Here's how the part is built. I have some questions about the finished solid (model axes, mm). Face numbers are marked on the shaded views. A direction names the side the tool comes from. Give positions to 0.01 mm unless a question says otherwise; leave off trailing zeros. Loops run counter-clockwise (first coordinate to the right, second up) from the corner with the lowest first, then second, coordinate; pieces in that order, holes last.
Q1. If we section it at A-A (x = 15): Please give me the cut outline in (y, z), plus the area to 3 significant figures.
Q2. I need wall thicknesses on line 1 (Y direction, x = 0, z = -38); line 2 (Y direction, x = -0.5, z = -27); line 3 (Y direction, x = -32.5, z = -31.5). Which ranges of each line are inside material? Lowest first, please.
Q3. If we section it at C-C (z = -11): Please give me the cut outline in (x, y), plus the area to 3 significant figures.
Q4. If we section it at D-D (x = 0): Give the number of separate pieces and of enclosed holes in the cut face, plus the area to 3 significant figures.
Q5. If we section it at B-B (z = -26): Please give me the cut outline in (x, y).
Q6. Will these pins go through, and if not, where does the flat tip stop? P1, Ø1, axis at x = -25, y = 13.5, coming from the -Z side; P2, Ø9, axis at x = 6.47, y = 42.54, coming from the -Z side; P3, Ø1.9, axis at y = 102.5, z = -41, coming from the +X side.
Q7. For the marked faces 4, 5 and 6, which set-ups out of +Z, -Z, +X, -X, +Y, -Y let a thin tool reach every point of the face, with its end or its side?
Q8. We'd pull the mould along Y, two halves only. Please class the marked faces 1, 2 and 3: +Y half, -Y half, draft (parallel to the pull), parting line (faces both ways), or undercut.
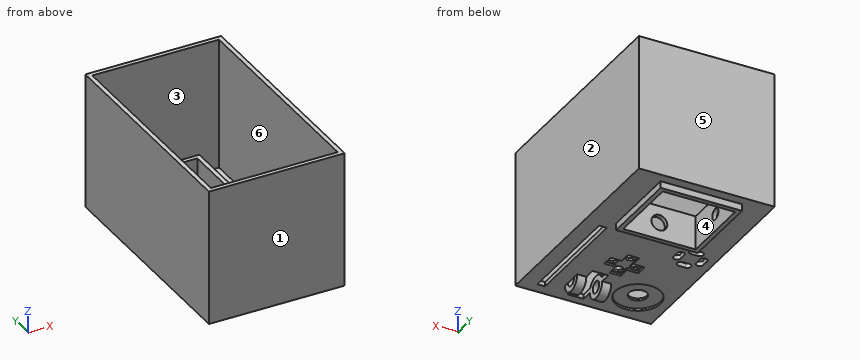
from build123d import *

# Parameters (mm, degrees)
SKETCH1_W                       = 76.2
SKETCH1_H                       = 76.2
BOX_DEPTH                       = 127
HOLLOW_IT_T                     = -2.54
SKETCH2_W                       = 4.318
SKETCH2_H                       = 63.5
SLIDER_TRACK_DEPTH              = 2.54
DPAD_LARGE_SHAPE_DEPTH          = 1.27
SKETCH7_R                       = 2.794
DPAD_TINY_HOLES_DEPTH           = 1.27
SKETCH8_R                       = 12.7
DIAL_LARGE_RING_DEPTH           = 1.27
SKETCH9_R                       = 5.08
DIAL_SMALL_HOLE_DEPTH           = 1.27
SKETCH12_W                      = 8.89
SKETCH12_H                      = 25.4
HOLE_FOR_SCROLL_WHEEL_DEPTH     = 2.54
SKETCH14_R                      = 6.35
NIBBLE_BASE_1_DEPTH             = 5.08
NIBBLE_START                    = -5.08
SKETCH15_R                      = 6.35
NIBBLE_BASE_2_DEPTH             = 5.08
NIBBLE_HOLES_REACH              = 145.381
SKETCH16_R                      = 3.302
NIBBLE_HOLES_DIRECTION_2_REACH  = 145.381
SINGLE_BUTTON_LEG_HOLE_DEPTH    = 2.54
MOAR_LEG_HOLES_COUNT            = 4
BASE_FOR_JOYSTICK_DEPTH         = 3.81
BASE_FOR_JOYSTICK_DEPTH_BACK    = 15.24
SKETCH19_W                      = 45.72
SKETCH19_H                      = 45.72
SKETCH21_W                      = 40.64
SKETCH21_H                      = 40.64
JOYSTICK_HOLE_DEPTH             = 155.861906549
LARGE_NIBBLES_REACH             = 148.689
SKETCH22_R                      = 3.175
LARGE_NIBBLES_DIRECTION_2_REACH = 148.689
SMALL_NIBBLES_REACH             = 134.524
SKETCH23_R                      = 4.445
SMALL_NIBBLES_DIRECTION_2_DEPTH = 48.26


with BuildPart() as part:
    # Sketch1 → box (new body)
    with BuildSketch(Plane(origin=(0, 0, 0), x_dir=(1, 0, 0), z_dir=(0, 1, 0))):
        Rectangle(SKETCH1_W, SKETCH1_H)
    extrude(amount=BOX_DEPTH)

    # hollow it
    hollow_it_openings = [part.faces().sort_by_distance(p)[0] for p in [
        (0, 63.5, 38.1),
    ]]
    offset(amount=HOLLOW_IT_T, openings=hollow_it_openings, kind=Kind.INTERSECTION)

    # Sketch2 → slider track (cut)
    with BuildSketch(Plane(origin=(0, 0, -38.1), x_dir=(-1, 0, 0), z_dir=(0, 0, -1))):
        with Locations((-27.051, 38.1)):
            Rectangle(SKETCH2_W, SKETCH2_H)
    extrude(amount=-SLIDER_TRACK_DEPTH, mode=Mode.SUBTRACT)

    # Sketch6 → dpad large shape (cut)
    with BuildSketch(Plane(origin=(0, 0, -38.1), x_dir=(-1, 0, 0), z_dir=(0, 0, -1))):
        Polygon((-3.297705804, 45.72), (-3.297705804, 52.07), (3.052294196, 52.07), (3.052294196, 45.72), (9.402294196, 45.72), (9.402294196, 39.37), (3.052294196, 39.37), (3.052294196, 33.02), (-3.297705804, 33.02), (-3.297705804, 39.37), (-9.647705804, 39.37), (-9.647705804, 45.72), align=None)
    extrude(amount=-DPAD_LARGE_SHAPE_DEPTH, mode=Mode.SUBTRACT)

    # Sketch7 → dpad tiny holes (cut)
    with BuildSketch(Plane(origin=(0, 0, -36.83), x_dir=(-1, 0, 0), z_dir=(0, 0, -1))):
        with Locations((-0.122705804, 48.895)):
            Circle(SKETCH7_R)
        with Locations((6.227294196, 42.672)):
            Circle(SKETCH7_R)
        with Locations((-0.122705804, 36.195)):
            Circle(SKETCH7_R)
        with Locations((-6.472705804, 42.545)):
            Circle(SKETCH7_R)
    extrude(amount=-DPAD_TINY_HOLES_DEPTH, mode=Mode.SUBTRACT)

    # Sketch8 → dial large ring (cut)
    with BuildSketch(Plane(origin=(0, 0, -38.1), x_dir=(-1, 0, 0), z_dir=(0, 0, -1))):
        with Locations((20.32, 19.05)):
            Circle(SKETCH8_R)
    extrude(amount=-DIAL_LARGE_RING_DEPTH, mode=Mode.SUBTRACT)

    # Sketch9 → dial small hole (cut)
    with BuildSketch(Plane(origin=(0, 0, -36.83), x_dir=(-1, 0, 0), z_dir=(0, 0, -1))):
        with Locations((20.32, 19.05)):
            Circle(SKETCH9_R)
    extrude(amount=-DIAL_SMALL_HOLE_DEPTH, mode=Mode.SUBTRACT)

    # Sketch12 → hole for scroll wheel (cut)
    with BuildSketch(Plane(origin=(0, 0, -38.1), x_dir=(-1, 0, 0), z_dir=(0, 0, -1))):
        with Locations((-6.985, 17.78)):
            Rectangle(SKETCH12_W, SKETCH12_H)
    extrude(amount=-HOLE_FOR_SCROLL_WHEEL_DEPTH, mode=Mode.SUBTRACT)

    # Sketch14 → nibble base 1 (add)
    with BuildSketch(Plane(origin=(2.54, 0, 0), x_dir=(0, 0, -1), z_dir=(1, 0, 0))):
        with Locations((38.1, 17.78)):
            Circle(SKETCH14_R)
    extrude(amount=-NIBBLE_BASE_1_DEPTH)

    # Sketch15 → nibble base 2 (add)
    with BuildSketch(Plane.ZY.offset(-11.43).offset(NIBBLE_START)):
        with Locations((-38.1, 17.78)):
            Circle(SKETCH15_R)
    extrude(amount=NIBBLE_BASE_2_DEPTH)

    # nibble holes: up to this face of the body (flat: up to its plane)
    nibble_holes_end = Plane(part.part.faces().sort_by_distance((16.51, 17.78, -40.795023703))[0])
    # Sketch16 → nibble holes (cut, up to the picked face)
    with BuildSketch(Plane.ZY.offset(-11.43), mode=Mode.PRIVATE) as nibble_holes_sk1:
        with Locations(Location((-38.1, 17.78, 0), (0, 0, 90))):
            Circle(SKETCH16_R)
    nibble_holes_tool1 = split(extrude(nibble_holes_sk1.sketch, amount=-NIBBLE_HOLES_REACH, mode=Mode.PRIVATE), bisect_by=nibble_holes_end, keep=Keep.BOTH, mode=Mode.PRIVATE)
    add(nibble_holes_tool1.solids().sort_by(Axis((11.43, 17.78, -38.1), (1, 0, 0)))[0], mode=Mode.SUBTRACT)

    # nibble holes direction 2: up to this face of the body (flat: up to its plane)
    nibble_holes_direction_2_end = Plane(part.part.faces().sort_by_distance((-2.54, 17.78, -40.795023703))[0])
    # Sketch16 → nibble holes direction 2 (cut, up to the picked face)
    with BuildSketch(Plane.ZY.offset(-11.43), mode=Mode.PRIVATE) as nibble_holes_direction_2_sk1:
        with Locations(Location((-38.1, 17.78, 0), (0, 0, 90))):
            Circle(SKETCH16_R)
    nibble_holes_direction_2_tool1 = split(extrude(nibble_holes_direction_2_sk1.sketch, amount=NIBBLE_HOLES_DIRECTION_2_REACH, mode=Mode.PRIVATE), bisect_by=nibble_holes_direction_2_end, keep=Keep.BOTH, mode=Mode.PRIVATE)
    add(nibble_holes_direction_2_tool1.solids().sort_by(Axis((11.43, 17.78, -38.1), (-1, 0, 0)))[0], mode=Mode.SUBTRACT)

    # Sketch17 → single button leg hole (cut)
    with BuildSketch(Plane(origin=(0, 0, -38.1), x_dir=(-1, 0, 0), z_dir=(0, 0, -1))):
        with BuildLine():
            Line((33.782, 65.405), (33.782, 61.595))
            ThreePointArc((33.782, 61.595), (31.75, 59.563), (29.718, 61.595))
            Line((29.718, 61.595), (29.718, 65.405))
            ThreePointArc((29.718, 65.405), (31.75, 67.437), (33.782, 65.405))
        make_face()
    single_button_leg_hole = extrude(amount=-SINGLE_BUTTON_LEG_HOLE_DEPTH, mode=Mode.SUBTRACT)

    # moar leg holes: single button leg hole ×4 about axis
    moar_leg_holes_axis = Axis((-25.4, 63.5, 0), (0, 0, 1))
    for i in range(1, MOAR_LEG_HOLES_COUNT):
        add(single_button_leg_hole.rotate(moar_leg_holes_axis, i * 360 / MOAR_LEG_HOLES_COUNT), mode=Mode.SUBTRACT)

    # Sketch19 → base for joystick (add, two sides: drawn at the far end of the back side and taken through both)
    with BuildSketch(Plane(origin=(0, 0, -38.1), x_dir=(-1, 0, 0), z_dir=(0, 0, -1)).offset(-BASE_FOR_JOYSTICK_DEPTH_BACK)):
        with Locations((0, 98.571636182)):
            Rectangle(SKETCH19_W, SKETCH19_H)
    extrude(amount=BASE_FOR_JOYSTICK_DEPTH + BASE_FOR_JOYSTICK_DEPTH_BACK)

    # Sketch21 → joystick hole (cut, through all)
    with BuildSketch(Plane(origin=(0, 0, -41.91), x_dir=(-1, 0, 0), z_dir=(0, 0, -1))):
        with Locations((0, 98.571636182)):
            Rectangle(SKETCH21_W, SKETCH21_H)
    extrude(amount=-JOYSTICK_HOLE_DEPTH, mode=Mode.SUBTRACT)

    # large nibbles: up to this face of the body (flat: up to its plane)
    large_nibbles_end = Plane(part.part.faces().sort_by_distance((-22.86, 98.571636182, -40.005))[0])
    # Sketch22 → large nibbles (cut, up to the picked face)
    with BuildSketch(Plane(origin=(-20.32, 0, 0), x_dir=(0, 0, -1), z_dir=(1, 0, 0)), mode=Mode.PRIVATE) as large_nibbles_sk1:
        with Locations((32.385, 98.571636182)):
            Circle(SKETCH22_R)
    large_nibbles_tool1 = split(extrude(large_nibbles_sk1.sketch, amount=-LARGE_NIBBLES_REACH, mode=Mode.PRIVATE), bisect_by=large_nibbles_end, keep=Keep.BOTH, mode=Mode.PRIVATE)
    add(large_nibbles_tool1.solids().sort_by(Axis((-20.32, 98.571636, -32.385), (-1, 0, 0)))[0], mode=Mode.SUBTRACT)

    # large nibbles direction 2: up to this face of the body (flat: up to its plane)
    large_nibbles_direction_2_end = Plane(part.part.faces().sort_by_distance((22.86, 98.571636182, -40.005))[0])
    # Sketch22 → large nibbles direction 2 (cut, up to the picked face)
    with BuildSketch(Plane(origin=(-20.32, 0, 0), x_dir=(0, 0, -1), z_dir=(1, 0, 0)), mode=Mode.PRIVATE) as large_nibbles_direction_2_sk1:
        with Locations((32.385, 98.571636182)):
            Circle(SKETCH22_R)
    large_nibbles_direction_2_tool1 = split(extrude(large_nibbles_direction_2_sk1.sketch, amount=LARGE_NIBBLES_DIRECTION_2_REACH, mode=Mode.PRIVATE), bisect_by=large_nibbles_direction_2_end, keep=Keep.BOTH, mode=Mode.PRIVATE)
    add(large_nibbles_direction_2_tool1.solids().sort_by(Axis((-20.32, 98.571636, -32.385), (1, 0, 0)))[0], mode=Mode.SUBTRACT)

    # small nibbles: up to this face of the body (flat: up to its plane)
    small_nibbles_end = Plane(part.part.faces().sort_by_distance((0, 124.46, 1.27))[0])
    # Sketch23 → small nibbles (cut, up to the picked face)
    with BuildSketch(Plane.XZ.offset(-118.891636182), mode=Mode.PRIVATE) as small_nibbles_sk1:
        with Locations(Location((0, -32.385, 0), (0, 0, 270))):
            Circle(SKETCH23_R)
    small_nibbles_tool1 = split(extrude(small_nibbles_sk1.sketch, amount=-SMALL_NIBBLES_REACH, mode=Mode.PRIVATE), bisect_by=small_nibbles_end, keep=Keep.BOTH, mode=Mode.PRIVATE)
    add(small_nibbles_tool1.solids().sort_by(Axis((0, 118.891636, -32.385), (0, 1, 0)))[0], mode=Mode.SUBTRACT)

    # Sketch23 → small nibbles direction 2 (cut)
    with BuildSketch(Plane.XZ.offset(-118.891636182)):
        with Locations(Location((0, -32.385, 0), (0, 0, 270))):
            Circle(SKETCH23_R)
    extrude(amount=SMALL_NIBBLES_DIRECTION_2_DEPTH, mode=Mode.SUBTRACT)


solid = part.part
Check sheet entries:
1. outline: (0, -38.1) - (11.43, -38.1) arc R6.35 ccw to (24.13, -38.1) - (75.71, -38.1) - (75.71, -41.91) - (78.25, -41.91) - (78.25, -22.86) - (75.71, -22.86) - (75.71, -35.56) - (23.6, -35.56) arc R6.35 ccw to (11.96, -35.56) - (2.54, -35.56) - (2.54, 38.1) - (0, 38.1) - close; (118.89, -41.91) - (121.43, -41.91) - (121.43, -38.1) - (127, -38.1) - (127, 38.1) - (124.46, 38.1) - (124.46, -35.56) - (121.43, -35.56) - (121.43, -22.86) - (118.89, -22.86) - close; hole circle Ø6.6 at (17.78, -38.1)
1. area: 738 mm2
2. line 1: y = 0 to 14.48, 21.08 to 33.02, 52.07 to 78.25, 118.89 to 127
2. line 2: y = 0 to 2.54, 75.71 to 78.25, 118.89 to 121.43, 124.46 to 127
2. line 3: y = 0 to 2.54, 124.46 to 127
3. outline: (-38.1, 0) - (38.1, 0) - (38.1, 127) - (-38.1, 127) - close; hole (-35.56, 2.54) - (35.56, 2.54) - (35.56, 124.46) - (-35.56, 124.46) - close
3. area: 1,010 mm2
4. separate pieces: 6
4. enclosed holes: 1
4. area: 645 mm2
5. outline: (-38.1, 0) - (38.1, 0) - (38.1, 127) - (-38.1, 127) - close; (-22.86, 75.71) - (22.86, 75.71) - (22.86, 121.43) - (-22.86, 121.43) - close; hole (-35.56, 2.54) - (35.56, 2.54) - (35.56, 124.46) - (-35.56, 124.46) - close; hole (-20.32, 78.25) - (20.32, 78.25) - (20.32, 118.89) - (-20.32, 118.89) - close
6. P1: stops at z = -36.83
6. P2: stops at z = -38.1
6. P3: stops at x = 22.86
7. face 4: +Z, -Z
7. face 5: +Z, -Z, +X, -X, +Y
7. face 6: +Z
8. face 1: -Y half
8. face 2: draft
8. face 3: undercut
